Build history of the part. All positions in model axes, mm. A direction names the side the tool comes from. Coordinates: 2 decimals unless noted, no trailing zeros. Order: outer loops, then holes, each group sorted by start corner. A loop starts at its lowest first (then second) coordinate and runs counter-clockwise, first axis right, second up. Notation, with made-up numbers: (-12.75, -23) - (11.25, -23) arc R21 cw to (11.25, 13) - close; hole circle Ø5 at (49, 78). An arc over 180 degrees is marked (long way). Return JSON: item names as keys, results as strings.
from build123d import *

# Parameters (mm, degrees)
SKETCH2_R           = 2.5
BOSS_EXTRUDE1_DEPTH = 14
SKETCH3_R           = 8
BOSS_EXTRUDE2_DEPTH = 8
SKETCH4_R           = 2.5
CUT_EXTRUDE1_DEPTH  = 23
CHAMFER1_SIZE       = 1


with BuildPart() as part:
    # Sketch2 → Boss-Extrude1 (new body)
    with BuildSketch(Plane.XY):
        Polygon((4.873707771, 0), (4.832012177, -0.636146486), (4.707640171, -1.261407971), (4.502718925, -1.865087032), (5.52904892, -2.817190886), (5.281517029, -3.257688046), (4.998967171, -3.676585913), (4.683272839, -4.071106911), (3.44623208, -3.44623208), (2.966924906, -3.866571903), (2.436853886, -4.2207551), (1.865087032, -4.502718925), (1.917572975, -5.901682854), (1.431063056, -6.038129807), (0.935064673, -6.134541988), (0.432866603, -6.190280914), (0, -4.873707771), (-0.636146486, -4.832012177), (-1.261407971, -4.707640171), (-1.865087032, -4.502718925), (-2.817190886, -5.52904892), (-3.257688046, -5.281517029), (-3.676585913, -4.998967171), (-4.071106911, -4.683272839), (-3.44623208, -3.44623208), (-3.866571903, -2.966924906), (-4.2207551, -2.436853886), (-4.502718925, -1.865087032), (-5.901682854, -1.917572975), (-6.038129807, -1.431063056), (-6.134541988, -0.935064673), (-6.190280914, -0.432866603), (-4.873707771, 0), (-4.832012177, 0.636146486), (-4.707640171, 1.261407971), (-4.502718925, 1.865087032), (-5.52904892, 2.817190886), (-5.281517029, 3.257688046), (-4.998967171, 3.676585913), (-4.683272839, 4.071106911), (-3.44623208, 3.44623208), (-2.966924906, 3.866571903), (-2.436853886, 4.2207551), (-1.865087032, 4.502718925), (-1.917572975, 5.901682854), (-1.431063056, 6.038129807), (-0.935064673, 6.134541988), (-0.432866603, 6.190280914), (0, 4.873707771), (0.636146486, 4.832012177), (1.261407971, 4.707640171), (1.865087032, 4.502718925), (2.817190886, 5.52904892), (3.257688046, 5.281517029), (3.676585913, 4.998967171), (4.071106911, 4.683272839), (3.44623208, 3.44623208), (3.866571903, 2.966924906), (4.2207551, 2.436853886), (4.502718925, 1.865087032), (5.901682854, 1.917572975), (6.038129807, 1.431063056), (6.134541988, 0.935064673), (6.190280914, 0.432866603), align=None)
        Circle(SKETCH2_R, mode=Mode.SUBTRACT)
    extrude(amount=BOSS_EXTRUDE1_DEPTH)

    # Sketch3 → Boss-Extrude2 (add)
    with BuildSketch(Plane(origin=(0, 0, 0), x_dir=(-1, 0, 0), z_dir=(0, 0, -1))):
        Circle(SKETCH3_R)
    extrude(amount=BOSS_EXTRUDE2_DEPTH)

    # Sketch4 → Cut-Extrude1 (cut, through all)
    with BuildSketch(Plane(origin=(0, 0, -8), x_dir=(-1, 0, 0), z_dir=(0, 0, -1))):
        Circle(SKETCH4_R)
    extrude(amount=-CUT_EXTRUDE1_DEPTH, mode=Mode.SUBTRACT)

    # Chamfer1
    chamfer1_edges = [part.edges().sort_by_distance(p)[0] for p in [
        (8, 0, 0),
    ]]
    chamfer(chamfer1_edges, length=CHAMFER1_SIZE)


solid = part.part
1. Probe L1, parallel to Z at x = -2.25, y = -6; L2, parallel to Y at x = 3.5, z = 12.25; L3, parallel to X at y = -1, z = -4. List the from-to ranges inside material, lowest first.
Check values:
{"L1": "-8 to 0", "L2": "-3.47 to 3.38, 3.55 to 5.12", "L3": "-7.94 to -2.29, 2.29 to 7.94"}
2. Mould opens along Y. For faces 4 (the flat face through (2.334, 5.009, 6.902)), 5 (the flat face through (-2, 2, -8)), 6 (the flat face through (5.54, 0.22, 6.9)), 7 (the flat face through (-1.89, 5.19, 6.9)) say: pulls with the +Y half, pulls with the -Y half, needs draft (parallel to the pull), parting line crosses it, or undercut.
Check values:
{"face 4": "pulls with the +Y half", "face 5": "needs draft", "face 6": "undercut", "face 7": "undercut"}
3. Drop flat-ended pins along their axis: pin 1 (5 mm diameter, centred on x = 5, z = 1, fed in from +Y); pin 2 (3 mm diameter, centred on x = 0, y = 0, fed in from +Z); pin 3 (5 mm diameter, centred on y = -5, z = -2, fed in from +X); pin 4 (3 mm diameter, centred on x = -1.5, z = 3.5, fed in from -Y). Give the stop position or say it passes through.
Check values:
{"pin 1": "y = 7.19", "pin 2": "through", "pin 3": "x = 7.6", "pin 4": "y = -5.53"}
4. Cut at A-A on z = -2.5. Give the cut face in (x, y).
Check values:
{"outline": "circle Ø16 at (0, 0); hole circle Ø5 at (0, 0)"}
5. Tool access for faces 1 (the flat face through (3.76, 4.07, 6.9)), 2 (the flat face through (-0.22, 5.54, 6.9)), 3 (the flat face through (-5.009, 2.334, 6.902)): list every direction of +Z, -Z, +X, -X, +Y, -Y with a clear straight run to the whole face (end or side of a thin tool).
Check values:
{"face 1": "+Z, +X", "face 2": "+Z, +Y", "face 3": "+Z, -X"}
